```python
from build123d import *

# Parameters (mm, degrees)
F0_W     = 50.8
F0_H     = 101.6
F1_DEPTH = 1850
F2_W     = 50.8
F2_H     = 101.6
F3_DEPTH = 50
F4_W     = 25.4
F4_H     = 101.6
F5_DEPTH = 50.8


with BuildPart() as f1:
    # F0 (on Top) → F1 (new body)
    with BuildSketch(Plane.XY):
        Rectangle(F0_W, F0_H)
    extrude(amount=F1_DEPTH)

    # F2 (on Right) → F3 (cut, symmetric)
    with BuildSketch(Plane.YZ):
        with Locations((25.4, 1449.2)):
            Rectangle(F2_W, F2_H)
    extrude(amount=F3_DEPTH, both=True, mode=Mode.SUBTRACT)

    # F4 (on face) → F5 (cut)
    with BuildSketch(Plane.XY.offset(1850)):
        with Locations((12.7, 0)):
            Rectangle(F4_W, F4_H)
    extrude(amount=-F5_DEPTH, mode=Mode.SUBTRACT)


solid = f1.part
```
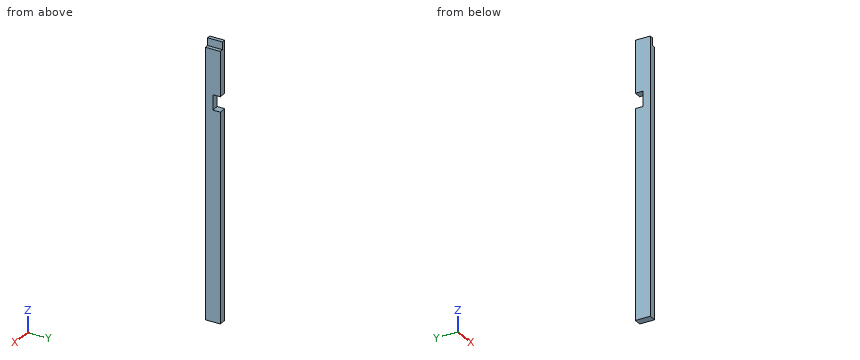
Geometry check sheet. Reference: the model listing, model coordinates, mm. Give positions to 0.01 mm unless a question says otherwise; leave off trailing zeros. Loops run counter-clockwise (first coordinate to the right, second up) from the corner with the lowest first, then second, coordinate; pieces in that order, holes last. Notation, with made-up numbers: M -18,85.25 L 18,85.25 A19 ccw 18,107.25 Z; hole C 14,-6.75 d2. An arc over 180 degrees is marked long. Answer as CSV lines item,"result".
Item 1: Cross-section at A-A on x = -12.5. Record the cut outline in (y, z).
Values:
outline,"M -50.8,0 L 50.8,0 L 50.8,1398.4 L 0,1398.4 L 0,1500 L 50.8,1500 L 50.8,1850 L -50.8,1850 Z"
Item 2: Depth check by flat-ended pin: P1, Ø1, axis at x = 11.5, y = -37.5, coming from the +Z side. Enter the tip coordinate at first touch or a pass-through.
Values:
P1,"stops at z = 1799.2"
Item 3: Material ranges on line 1 (Z direction, x = 6, y = 17.5); line 2 (Z direction, x = -4.5, y = 13.5); line 3 (Z direction, x = 4.5, y = -15), recorded low to high.
Values:
line 1,"z = 0 to 1398.4, 1500 to 1799.2"
line 2,"z = 0 to 1398.4, 1500 to 1850"
line 3,"z = 0 to 1799.2"
